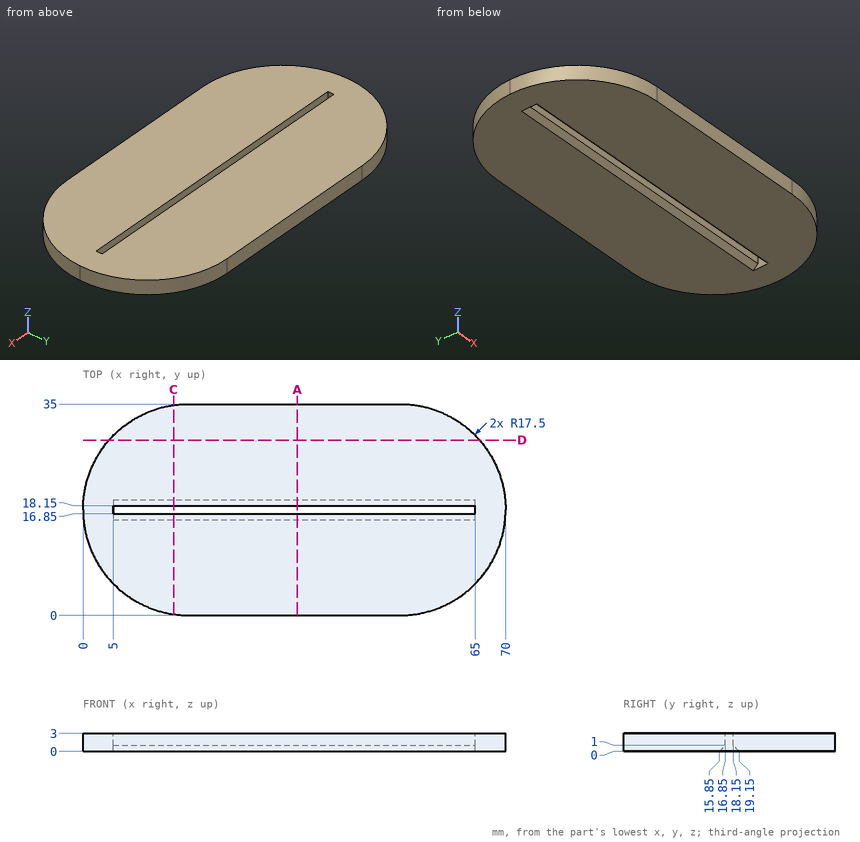
The drawing under review shows one solid part. Ordinate dimensions are in mm from its lowest x, y, z. Round coordinates to 2 decimals unless told otherwise and drop trailing zeros. Loops run counter-clockwise (first coordinate to the right, second up) from the corner with the lowest first, then second, coordinate; pieces in that order, holes last. Notation, with made-up numbers: (48.25, 32.5) - (78.25, 32.5) arc R11 cw to (78.25, 46.5) - close; hole circle Ø8 at (-35, 83). An arc over 180 degrees is marked (long way). Put each result on its own line as item: value. Start each with the question number.
1. Consider section C-C on x = 15. State the section outline as (y, z) points.
2. Consider section D-D on y = 29. State the section outline as (x, z) points.
3. Consider section A-A on x = 35.5. State the section outline as (y, z) points.
4. Insertion check: P1, Ø1.5, axis at y = 13.5, z = 2.5, coming from the +X side. The pin has a flat end and moves straight along its axis. Give the tip position at first contact, or say it passes through.
5. For probe 1 along Y at (x, z) = (20.5, 2.6); probe 2 along X at (y, z) = (18, 0.7); probe 3 along Y at (x, z) = (16, 1.05), list the stretches that pass through material, from the lowest coordinate up. Write a range as [from, to].
Result sheet:
1. outline: (0.18, 0) - (15.85, 0) - (16.85, 1) - (16.85, 3) - (0.18, 3) - close; (18.15, 1) - (19.15, 0) - (34.82, 0) - (34.82, 3) - (18.15, 3) - close
2. outline: (4.31, 0) - (65.69, 0) - (65.69, 3) - (4.31, 3) - close
3. outline: (0, 0) - (15.85, 0) - (16.85, 1) - (16.85, 3) - (0, 3) - close; (18.15, 1) - (19.15, 0) - (35, 0) - (35, 3) - (18.15, 3) - close
4. P1: x = 69.7
5. probe 1: [0, 16.85], [18.15, 35]
5. probe 2: [0.01, 5], [65, 69.99]
5. probe 3: [0.06, 16.85], [18.15, 34.94]
